Work out the finished part from the listing and answer in its coordinate system (mm). Round coordinates to 2 decimals unless told otherwise and drop trailing zeros. Write each loop counter-clockwise with the first axis right and the second up, starting at its lowest first coordinate (ties: lowest second). Pieces come first, ordered by that corner, then holes. Notation, with made-up numbers: (34, 56.25) -> (49, 56.25) arc R12 cw to (49, 78.25) -> close; hole circle Ø4 at (38.5, 26.25). An arc over 180 degrees is marked (long way). One line per item, written item: value.
```python
from build123d import *

# Parameters (mm, degrees)
F1_DEPTH = 6.35
F2_D     = 8.3312
F3_D     = 8.3312
F4_D     = 8.3312
F5_D     = 8.3312
F6_D     = 8.3312
F7_D     = 8.3312
F8_D     = 8.3312
F9_D     = 8.3312


with BuildPart() as f1:
    # F0 (on Front) → F1 (new body)
    with BuildSketch(Plane.XZ):
        Polygon((76.2, 57.15), (-76.2, 57.15), (-76.2, 19.05), (-50.8, -57.15), (50.8, -57.15), (76.2, 19.05), align=None)
    extrude(amount=F1_DEPTH)

    # F2 (through all)
    with Locations(Plane(origin=(0, 0, 0), x_dir=(1, 0, 0), z_dir=(0, 1, 0))):
        with Locations((57.15, -38.1)):
            Hole(F2_D / 2)

    # F3 (through all)
    with Locations(Plane(origin=(0, 0, 0), x_dir=(1, 0, 0), z_dir=(0, 1, 0))):
        with Locations((19.05, -38.1)):
            Hole(F3_D / 2)

    # F4 (through all)
    with Locations(Plane(origin=(0, 0, 0), x_dir=(1, 0, 0), z_dir=(0, 1, 0))):
        with Locations((-19.05, -38.1)):
            Hole(F4_D / 2)

    # F5 (through all)
    with Locations(Plane(origin=(0, 0, 0), x_dir=(1, 0, 0), z_dir=(0, 1, 0))):
        with Locations((-57.15, -38.1)):
            Hole(F5_D / 2)

    # F6 (through all)
    with Locations(Plane(origin=(0, 0, 0), x_dir=(1, 0, 0), z_dir=(0, 1, 0))):
        with Locations((-19.05, 0)):
            Hole(F6_D / 2)

    # F7 (through all)
    with Locations(Plane(origin=(0, 0, 0), x_dir=(1, 0, 0), z_dir=(0, 1, 0))):
        with Locations((19.05, 0)):
            Hole(F7_D / 2)

    # F8 (through all)
    with Locations(Plane(origin=(0, 0, 0), x_dir=(1, 0, 0), z_dir=(0, 1, 0))):
        with Locations((-19.05, 38.1)):
            Hole(F8_D / 2)

    # F9 (through all)
    with Locations(Plane(origin=(0, 0, 0), x_dir=(1, 0, 0), z_dir=(0, 1, 0))):
        with Locations((19.05, 38.1)):
            Hole(F9_D / 2)


solid = f1.part
```
(1) Find section A-A on z = -38.1. Give the vertices of the cut face in (x, y), plus the area to 3 significant figures.
Reported:
outline: (-57.15, -6.35) -> (-23.22, -6.35) -> (-23.22, 0) -> (-57.15, 0) -> close; (-14.88, -6.35) -> (14.88, -6.35) -> (14.88, 0) -> (-14.88, 0) -> close; (23.22, -6.35) -> (57.15, -6.35) -> (57.15, 0) -> (23.22, 0) -> close
area: 620 mm2
(2) Consider probe 1 along Z at (x, y) = (19.05, -4.5); probe 2 along X at (y, z) = (-2.75, 38.1); probe 3 along X at (y, z) = (-4.5, -38.1). Determine where each line is inside the solid, lowest interval first.
Reported:
probe 1: z = -57.15 to -42.27, -33.93 to -4.17, 4.17 to 33.93, 42.27 to 57.15
probe 2: x = -76.2 to -61.32, -52.98 to -23.22, -14.88 to 14.88, 23.22 to 52.98, 61.32 to 76.2
probe 3: x = -57.15 to -23.22, -14.88 to 14.88, 23.22 to 57.15
(3) For a pull along Z with two mould halves and no side action, classify faces 1 (the face through (63.322, -3.131, -19.583)), 2 (the face through (1, -3, 57.15)), 3 (the face through (23.21, -3.22, 37.92)), 4 (the face through (-52.99, -3.22, 37.92)) as pulls with the +Z half, pulls with the -Z half, needs draft (parallel to the pull), parting line crosses it, or undercut.
Reported:
face 1: pulls with the -Z half
face 2: pulls with the +Z half
face 3: undercut
face 4: undercut
(4) A flat-ended cylindrical pin translates along its axis: pin 1 Ø2 at (y, z) = (-2, -26.5) entering from +X. Find the tip coordinate at first contact, or state that the pin passes through.
Reported:
pin 1: stops at x = 61.35
(5) Find section D-D on x = -57.15. Give the vertices of the cut face in (y, z).
Reported:
outline: (-6.35, -38.1) -> (0, -38.1) -> (0, 33.93) -> (-6.35, 33.93) -> close; (-6.35, 42.27) -> (0, 42.27) -> (0, 57.15) -> (-6.35, 57.15) -> close
(6) Find section B-B on x = -19.05. Give the vertices of the cut face in (y, z).
Reported:
outline: (-6.35, -57.15) -> (0, -57.15) -> (0, -42.27) -> (-6.35, -42.27) -> close; (-6.35, -33.93) -> (0, -33.93) -> (0, -4.17) -> (-6.35, -4.17) -> close; (-6.35, 4.17) -> (0, 4.17) -> (0, 33.93) -> (-6.35, 33.93) -> close; (-6.35, 42.27) -> (0, 42.27) -> (0, 57.15) -> (-6.35, 57.15) -> close
(7) Find section C-C on y = -1.5. Give the number of separate pieces and of enclosed holes in the cut face, plus the area to 3 significant figures.
Reported:
separate pieces: 1
enclosed holes: 8
area: 15,000 mm2
